Geometry check sheet. Reference: the model listing, model coordinates, mm. A direction names the side the tool comes from. Give positions to 0.01 mm unless a question says otherwise; leave off trailing zeros. Loops run counter-clockwise (first coordinate to the right, second up) from the corner with the lowest first, then second, coordinate; pieces in that order, holes last. Notation, with made-up numbers: (42.25, 15.25) -> (84.25, 15.25) arc R8 cw to (84.25, 23.25) -> close; hole circle Ø9 at (64.25, 46.5). An arc over 180 degrees is marked (long way). Answer in a Markdown table with one row per item. Add a question column.
```python
from build123d import *

# Parameters (mm, degrees)
SKETCH1_R           = 12.5
BOSS_EXTRUDE1_DEPTH = 9
SKETCH2_R           = 8
BOSS_EXTRUDE2_DEPTH = 96
SKETCH4_R           = 1.5
CUT_EXTRUDE1_DEPTH  = 96


with BuildPart() as part:
    # Sketch1 → Boss-Extrude1 (new body)
    with BuildSketch(Plane(origin=(0, 0, 0), x_dir=(0, 0, -1), z_dir=(1, 0, 0))):
        Circle(SKETCH1_R)
    extrude(amount=BOSS_EXTRUDE1_DEPTH)

    # Sketch2 → Boss-Extrude2 (add)
    with BuildSketch(Plane(origin=(9, 0, 0), x_dir=(0, 0, -1), z_dir=(1, 0, 0))):
        Circle(SKETCH2_R)
    extrude(amount=BOSS_EXTRUDE2_DEPTH)

    # Sketch4 → Cut-Extrude1 (cut)
    with BuildSketch(Plane.XY.offset(8)):
        with Locations((98, 0)):
            Circle(SKETCH4_R)
    extrude(amount=-CUT_EXTRUDE1_DEPTH, mode=Mode.SUBTRACT)


solid = part.part
```
1. Access from +Z, -Z, +X, -X, +Y, -Y to the whole of each face (thin tool, end or side, straight path). Record for faces 1 (the face through (0, 0, 0)), 2 (the face through (9, -8.2, 0.2)).
2. Sectioned sample at C-C (x = 98). Enter the section's corners in (y, z), plus the area to 3 significant figures.
3. Sectioned sample at B-B (z = -2). Enter the section's corners in (x, y), plus the area to 3 significant figures.
4. Material ranges on L1, parallel to X at y = 0.25, z = -1.75; L2, parallel to X at y = -0.75, z = 9; L3, parallel to Y at x = 98, z = -2, recorded low to high. Write a range as from..to.
5. Sectioned sample at A-A (y = 0). Enter the section's corners in (x, z), plus the area to 3 significant figures.
6. Gauge pin test, flat ends, axial feed: pin 1 Ø10 at (x, y) = (94.5, -6.5) entering from -Z; pin 2 Ø6 at (x, z) = (86, -2) entering from +Y; pin 3 Ø6 at (x, z) = (28, -5) entering from -Y; pin 4 Ø2.5 at (x, y) = (98, 0) entering from +Z. Record the tip position at first contact, or that the pin passes through.
7. Sectioned sample at D-D (y = 4). Enter the section's corners in (x, z), plus the area to 3 significant figures.
Response:
| question | item | result |
|---|---|---|
| 1 | face 1 | +Z, -Z, -X, +Y, -Y |
| 1 | face 2 | +X |
| 2 | outline | (-1.5, -7.86) -> (-1.5, 7.86) arc R8 ccw to start; (1.5, -7.86) arc R8 ccw to (1.5, 7.86) -> close |
| 2 | area | 153 mm2 |
| 3 | outline | (0, -12.34) -> (9, -12.34) -> (9, -7.75) -> (105, -7.75) -> (105, 7.75) -> (9, 7.75) -> (9, 12.34) -> (0, 12.34) -> close; hole circle Ø3 at (98, 0) |
| 3 | area | 1,700 mm2 |
| 4 | L1 | x = 0..96.52, 99.48..105 |
| 4 | L2 | x = 0..9 |
| 4 | L3 | y = -7.75..-1.5, 1.5..7.75 |
| 5 | outline | (0, -12.5) -> (9, -12.5) -> (9, -8) -> (96.5, -8) -> (96.5, 8) -> (9, 8) -> (9, 12.5) -> (0, 12.5) -> close; (99.5, -8) -> (105, -8) -> (105, 8) -> (99.5, 8) -> close |
| 5 | area | 1,710 mm2 |
| 6 | pin 1 | stops at z = -7.86 |
| 6 | pin 2 | stops at y = 8 |
| 6 | pin 3 | stops at y = -7.75 |
| 6 | pin 4 | passes through |
| 7 | outline | (0, -11.84) -> (9, -11.84) -> (9, -6.93) -> (105, -6.93) -> (105, 6.93) -> (9, 6.93) -> (9, 11.84) -> (0, 11.84) -> close |
| 7 | area | 1,540 mm2 |
